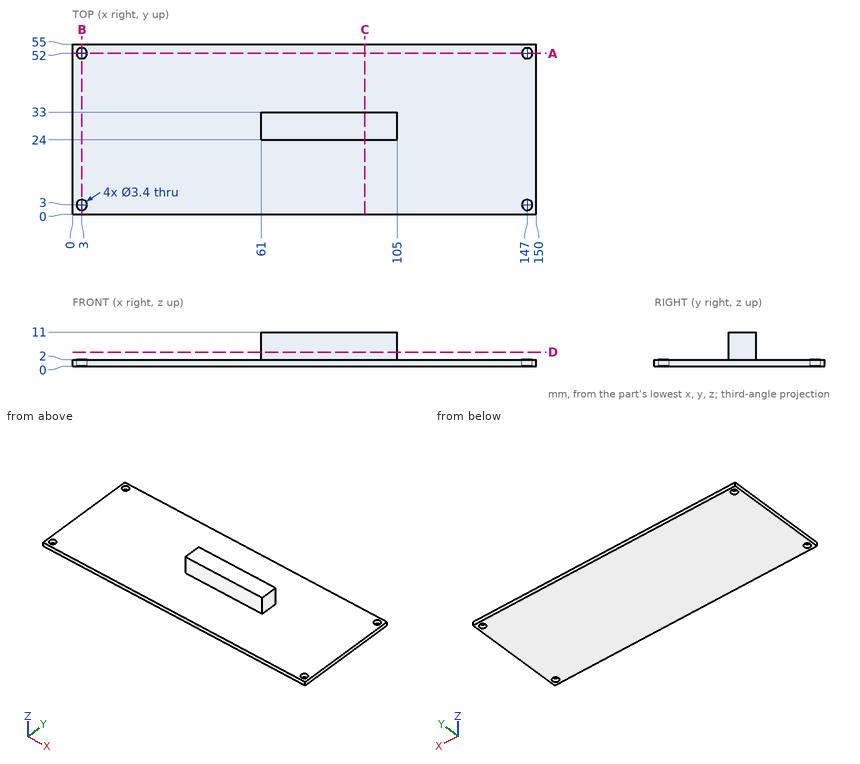
Check sheet for the drawn part. Datum: minimum x, y, z corner. Units: mm. Coordinates: 2 decimals unless noted, no trailing zeros. Order: outer loops, then holes, each group sorted by start corner. A loop starts at its lowest first (then second) coordinate and runs counter-clockwise, first axis right, second up. Notation, with made-up numbers: (-11, 76.25) - (23, 76.25) arc R20 cw to (23, 93.25) - close; hole circle Ø10 at (66, -4). An arc over 180 degrees is marked (long way). Return JSON: item names as keys, results as strings.
(1) Thickness scan on line 1 along Y through (x, z) = (147, 1.4); line 2 along Y through (x, z) = (74, 5.5); line 3 along Z through (x, y) = (124.5, 13.5). Record the ranges inside material, lowest first.
Filled sheet:
{"line 1": "y = 0 to 1.3, 4.7 to 50.3, 53.7 to 55", "line 2": "y = 24 to 33", "line 3": "z = 0 to 2"}
(2) Section check B-B, the plane x = 3. Record the cut outline in (y, z), and give its area (3 significant figures).
Filled sheet:
{"outline": "(0, 0) - (1.3, 0) - (1.3, 2) - (0, 2) - close; (4.7, 0) - (50.3, 0) - (50.3, 2) - (4.7, 2) - close; (53.7, 0) - (55, 0) - (55, 2) - (53.7, 2) - close", "area": "96.4 mm^2"}
(3) Section check C-C, the plane x = 94.5. Record the cut outline in (y, z).
Filled sheet:
{"outline": "(0, 0) - (55, 0) - (55, 2) - (33, 2) - (33, 11) - (24, 11) - (24, 2) - (0, 2) - close"}
(4) Section check D-D, the plane z = 4.5. Record the cut outline in (x, y).
Filled sheet:
{"outline": "(61, 24) - (105, 24) - (105, 33) - (61, 33) - close"}
(5) Go/stop test with flat-tipped pins: pin 1 (1 mm diameter, centred on x = 32, y = 26.5, fed in from +Z); pin 2 (4 mm diameter, centred on x = 82.5, z = 7, fed in from +Y); pin 3 (2 mm diameter, centred on x = 3, y = 52, fed in from -Z); pin 4 (2.5 mm diameter, centred on y = 28.5, z = 7, fed in from -X). Record where each tip stops, or that it passes through.
Filled sheet:
{"pin 1": "stops at z = 2", "pin 2": "stops at y = 33", "pin 3": "passes through", "pin 4": "stops at x = 61"}
(6) Section check A-A, the plane y = 52. Record the cut outline in (x, z).
Filled sheet:
{"outline": "(0, 0) - (1.3, 0) - (1.3, 2) - (0, 2) - close; (4.7, 0) - (145.3, 0) - (145.3, 2) - (4.7, 2) - close; (148.7, 0) - (150, 0) - (150, 2) - (148.7, 2) - close"}
